Print and shaded views of the part. All mm, measured from the part's lowest x, y and z. Coordinates: 2 decimals unless noted, no trailing zeros. Loops run counter-clockwise (first coordinate to the right, second up) from the corner with the lowest first, then second, coordinate; pieces in that order, holes last.
1) Saw through at A-A, the plane y = 6.5. Write the cut outline in (x, z).
2) Saw through at D-D, the plane y = 2.25. Write the cut outline in (x, z).
3) Two-plate mould, pull along Y, no slides. Class the marked faces 1 and 2: +Y half, -Y half, draft (parallel to the pull), parting line (faces both ways), or undercut.
4) Wall check: line 1 along X through (y, z) = (6.75, 0.65); line 2 along X through (y, z) = (6.25, 3.4); line 3 along Y through (x, z) = (9.25, 2.3) (1 decimal). Give the ranges that are in metal, low to high.
5) Saw through at C-C, the plane x = 6. Write the cut outline in (y, z), and give its area (3 significant figures).
6) Pin check, flat tips, straight feed: pin 1 Ø1 at (x, z) = (12.5, 0.5) entering from +Y; pin 2 Ø2 at (x, z) = (11, 1) entering from -Y; pin 3 Ø1 at (x, z) = (1.5, 1) entering from +Y. Stop position of each tip, or through.
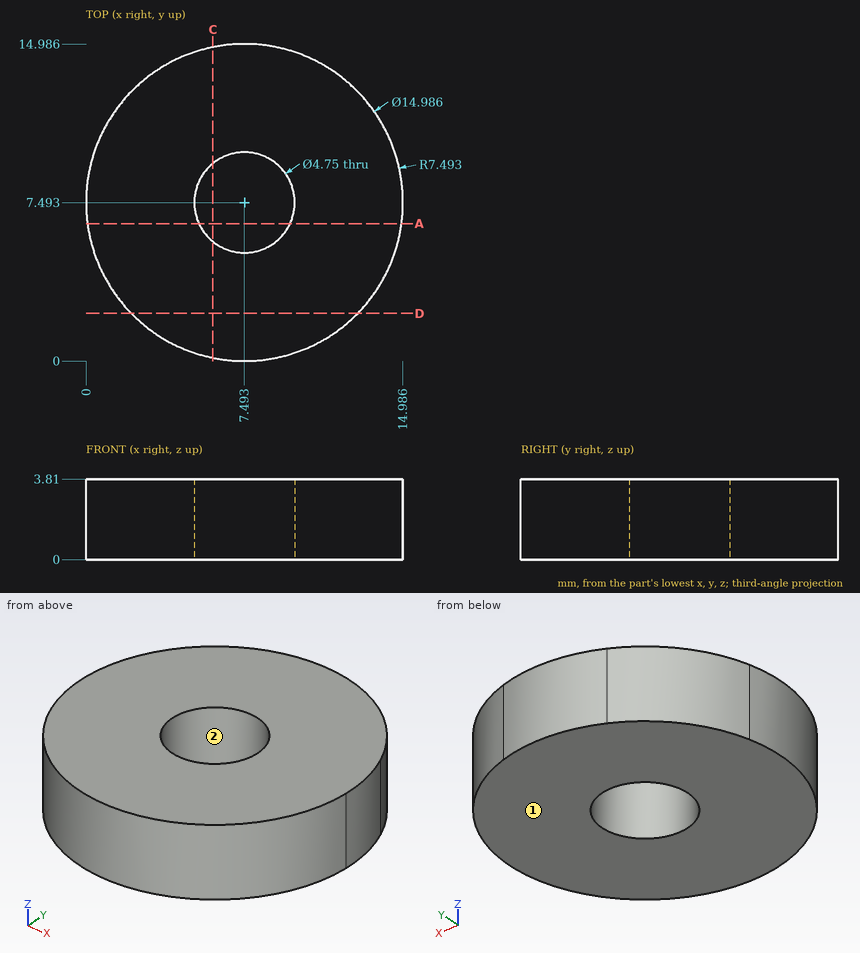
Data:
1. outline: (0.07, 0) - (5.34, 0) - (5.34, 3.81) - (0.07, 3.81) - close; (9.65, 0) - (14.92, 0) - (14.92, 3.81) - (9.65, 3.81) - close
2. outline: (2.14, 0) - (12.85, 0) - (12.85, 3.81) - (2.14, 3.81) - close
3. face 1: draft
3. face 2: undercut
4. line 1: x = 0.04 to 5.24, 9.75 to 14.95
4. line 2: x = 0.1 to 5.47, 9.52 to 14.88
4. line 3: y = 0.2 to 5.9, 9.1 to 14.8
5. outline: (0.15, 0) - (5.65, 0) - (5.65, 3.81) - (0.15, 3.81) - close; (9.34, 0) - (14.84, 0) - (14.84, 3.81) - (9.34, 3.81) - close
5. area: 41.9 mm2
6. pin 1: stops at y = 13.48
6. pin 2: stops at y = 0.43
6. pin 3: stops at y = 12.59
